Job drawing, mm, ordinate dimensions from the low corner. One solid piece. Give positions to 0.01 mm unless a question says otherwise; leave off trailing zeros. Loops run counter-clockwise (first coordinate to the right, second up) from the corner with the lowest first, then second, coordinate; pieces in that order, holes last.
Item 1: Probe probe 1 along X at (y, z) = (6.25, 2.1); probe 2 along X at (y, z) = (5.5, 1.2); probe 3 along Y at (x, z) = (45, 2.8) (1 decimal). List the from-to ranges inside material, lowest first.
Item 2: Drop flat-ended pins along their axis: P1, Ø1.4, axis at x = 47.625, y = 9.525, coming from the +Z side; P2, Ø1.8, axis at x = 44.6, y = 2.6, coming from the +Z side (3 decimals). Give the stop position or say it passes through.
Item 3: Saw through at B-B on y = 7.25. Give the cut face in (x, z) (1 decimal), plus the area to 3 significant figures.
Item 4: Saw through at C-C on z = 1.1. Give the number of separate pieces and of enclosed holes in the cut face.
Item 5: Saw through at A-A on x = 6.35. Give the cut face in (y, z) (3 decimals).
Item 6: Saw through at D-D on x = 38.1. Give the cut face in (y, z) (3 decimals).
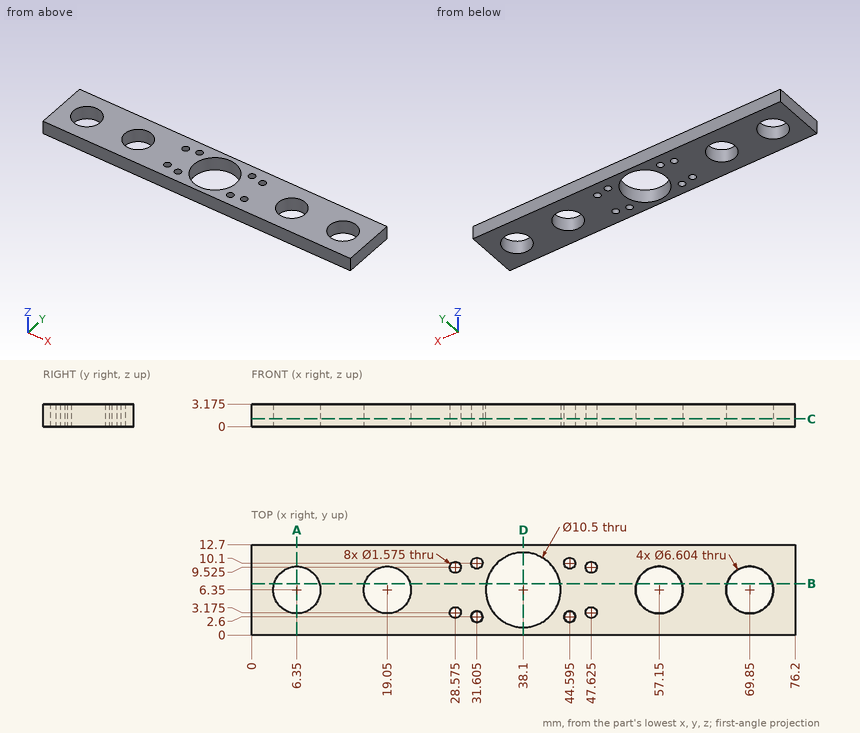
Results below:
1. probe 1: x = 0 to 3.05, 9.65 to 15.75, 22.35 to 32.85, 43.35 to 53.85, 60.45 to 66.55, 73.15 to 76.2
1. probe 2: x = 0 to 3.16, 9.54 to 15.86, 22.24 to 32.92, 43.28 to 53.96, 60.34 to 66.66, 73.04 to 76.2
1. probe 3: y = 0 to 1.9, 3.3 to 9.4, 10.8 to 12.7
2. P1: passes through
2. P2: stops at z = 3.175
3. outline: (0, 0) - (3.2, 0) - (3.2, 3.2) - (0, 3.2) - close; (9.5, 0) - (15.9, 0) - (15.9, 3.2) - (9.5, 3.2) - close; (22.2, 0) - (32.9, 0) - (32.9, 3.2) - (22.2, 3.2) - close; (43.3, 0) - (54, 0) - (54, 3.2) - (43.3, 3.2) - close; (60.3, 0) - (66.7, 0) - (66.7, 3.2) - (60.3, 3.2) - close; (73, 0) - (76.2, 0) - (76.2, 3.2) - (73, 3.2) - close
3. area: 128 mm2
4. separate pieces: 1
4. enclosed holes: 13
5. outline: (0, 0) - (3.048, 0) - (3.048, 3.175) - (0, 3.175) - close; (9.652, 0) - (12.7, 0) - (12.7, 3.175) - (9.652, 3.175) - close
6. outline: (0, 0) - (1.1, 0) - (1.1, 3.175) - (0, 3.175) - close; (11.6, 0) - (12.7, 0) - (12.7, 3.175) - (11.6, 3.175) - close
